from build123d import *

# Parameters (mm, degrees)
SKETCH1_W           = 118.75
SKETCH1_H           = 24
BOSS_EXTRUDE1_DEPTH = 10
SKETCH2_W           = 3.3
SKETCH2_H           = 9.8
BOSS_EXTRUDE2_DEPTH = 118.75
CUT_EXTRUDE1_REACH  = 123.333
SKETCH4_R           = 1.9
LPATTERN1_COUNT     = 5
LPATTERN1_PITCH     = 23.75


with BuildPart() as part:
    # Sketch1 → Boss-Extrude1 (new body)
    with BuildSketch(Plane.YZ):
        with Locations((59.375, 12)):
            Rectangle(SKETCH1_W, SKETCH1_H)
    extrude(amount=-BOSS_EXTRUDE1_DEPTH)

    # Sketch2 → Boss-Extrude2 (add, through all)
    with BuildSketch(Plane.XZ):
        with Locations((-5, -4.9)):
            Rectangle(SKETCH2_W, SKETCH2_H)
    extrude(amount=-BOSS_EXTRUDE2_DEPTH)

    # Sketch4 → Cut-Extrude1 (cut, up to next)
    with BuildSketch(Plane(origin=(-6.65, 0, 0), x_dir=(0, -1, 0), z_dir=(-1, 0, 0)), mode=Mode.PRIVATE) as cut_extrude1_sk1:
        with Locations(Location((-106.875, -5, 0), (0, 0, 90))):
            Circle(SKETCH4_R)
    cut_extrude1_tool1 = extrude(cut_extrude1_sk1.sketch, amount=-CUT_EXTRUDE1_REACH, mode=Mode.PRIVATE) & part.part
    cut_extrude1 = cut_extrude1_tool1.solids().sort_by_distance((-6.65, 106.875, -5))[0]
    add(cut_extrude1, mode=Mode.SUBTRACT)

    # LPattern1: Cut-Extrude1 ×5
    with Locations(*[(0, -i * LPATTERN1_PITCH, 0) for i in range(1, LPATTERN1_COUNT)]):
        add(cut_extrude1, mode=Mode.SUBTRACT)


solid = part.part
The listing builds one solid part. Answer for the finished solid, in the listing's coordinates (mm). A direction names the side the tool comes from. Coordinates: 2 decimals unless noted, no trailing zeros. Loops run counter-clockwise (first coordinate to the right, second up) from the corner with the lowest first, then second, coordinate; pieces in that order, holes last. Notation, with made-up numbers: M 36.25,3.5 L 55.25,3.5 A25 cw 55.25,16.5 Z; hole C -12,30.5 d4. An arc over 180 degrees is marked long. Answer in a Markdown table with one row per item.
1) Given pin 1 (3 mm diameter, centred on y = 11.875, z = -5, fed in from +X); pin 2 (3 mm diameter, centred on y = 84, z = -7, fed in from -X); pin 3 (1.7 mm diameter, centred on x = -1, y = 41.5, fed in from -Z); pin 4 (3 mm diameter, centred on y = 78.5, z = -6, fed in from +X), each flat-ended and moving along its own axis, determine where each tip first touches the part or whether it passes through.
Answers below:
| item | result |
|---|---|
| pin 1 | through |
| pin 2 | x = -6.65 |
| pin 3 | z = 0 |
| pin 4 | x = -3.35 |
2) Find section B-B (y = 8.5). Determine the outline of the cut face in (x, z).
Answers below:
| item | result |
|---|---|
| outline | M -10,0 L -6.65,0 L -6.65,-9.8 L -3.35,-9.8 L -3.35,0 L 0,0 L 0,24 L -10,24 Z |
3) Determine the mould class of faces 1 (the cylindrical face through (-5.02, 81.27, -5.41)), 2 (the flat face through (-8, 59, 0)), 3 (the flat face through (-5, 0, 11)), 4 (the flat face through (-5, 118.75, 11)) for opening direction Y: released by +Y, released by -Y, zero draft, split by the parting line, or undercut.
Answers below:
| item | result |
|---|---|
| face 1 | undercut |
| face 2 | zero draft |
| face 3 | released by -Y |
| face 4 | released by +Y |
4) Which of the six approach directions +Z, -Z, +X, -X, +Y, -Y give full straight-line access (tool end or side, diameter ignored) to faces 5 (the flat face through (-3.35, 58.5, -2.8)), 6 (the flat face through (-5, 59, -9.8)), 7 (the flat face through (-6.65, 58.5, -2.8))?
Answers below:
| item | result |
|---|---|
| face 5 | -Z, +X, +Y, -Y |
| face 6 | -Z, +X, -X, +Y, -Y |
| face 7 | -Z, -X, +Y, -Y |
5) Find section C-C (x = -8.5). Determine the outline of the cut face in (y, z).
Answers below:
| item | result |
|---|---|
| outline | M 0,0 L 118.75,0 L 118.75,24 L 0,24 Z |
6) Find the intervals of material crossed by probe 1 along Y at (x, z) = (-4.1, -5) (3 decimals); probe 2 along Z at (x, y) = (-7.25, 54); probe 3 along X at (y, z) = (22, -5), in increasing order.
Answers below:
| item | result |
|---|---|
| probe 1 | 0 to 9.975, 13.775 to 33.725, 37.525 to 57.475, 61.275 to 81.225, 85.025 to 104.975, 108.775 to 118.75 |
| probe 2 | 0 to 24 |
| probe 3 | -6.65 to -3.35 |
7) Find section A-A (z = -5). Determine the outline of the cut face in (x, y) (3 decimals), then the cut area to 3 significant figures.
Answers below:
| item | result |
|---|---|
| outline | M -6.65,0 L -3.35,0 L -3.35,9.975 L -6.65,9.975 Z; M -6.65,13.775 L -3.35,13.775 L -3.35,33.725 L -6.65,33.725 Z; M -6.65,37.525 L -3.35,37.525 L -3.35,57.475 L -6.65,57.475 Z; M -6.65,61.275 L -3.35,61.275 L -3.35,81.225 L -6.65,81.225 Z; M -6.65,85.025 L -3.35,85.025 L -3.35,104.975 L -6.65,104.975 Z; M -6.65,108.775 L -3.35,108.775 L -3.35,118.75 L -6.65,118.75 Z |
| area | 329 mm^2 |
